Source: CAD feature listing. Evaluate the final solid. Frame: model axes, mm. A direction names the side the tool comes from. Give positions to 0.01 mm unless a question says otherwise; leave off trailing zeros. Write each loop counter-clockwise with the first axis right and the second up, starting at its lowest first coordinate (ties: lowest second). Pieces come first, ordered by that corner, then holes. Notation, with made-up numbers: M -8,79 L 11,79 A8 cw 11,84 Z; hole C 35,43.5 d2. An arc over 180 degrees is marked long. Return JSON: item names as keys, results as strings.
```python
from build123d import *

# Parameters (mm, degrees)
F1_DEPTH = 360.3625
F2_R     = 3.175
F3_DEPTH = 9.525


with BuildPart() as f1:
    # F0 (on Front) → F1 (new body)
    with BuildSketch(Plane.XZ):
        Polygon((3.666174, 6.35), (-3.666174, 6.35), (-7.332348, 0), (-3.666174, -6.35), (3.666174, -6.35), (7.332348, 0), align=None)
    extrude(amount=F1_DEPTH)

    # F2 (on face) → F3 (cut)
    with BuildSketch(Plane(origin=(0, 0, 0), x_dir=(-1, 0, 0), z_dir=(0, 1, 0))):
        Circle(F2_R)
    extrude(amount=-F3_DEPTH, mode=Mode.SUBTRACT)


solid = f1.part
```
1) Cut plane A-A, the plane y = -59. Return the cut outline in (x, z), then the cut area to 3 significant figures.
Numbers:
{"outline": "M -7.33,0 L -3.67,-6.35 L 3.67,-6.35 L 7.33,0 L 3.67,6.35 L -3.67,6.35 Z", "area": "140 mm²"}
2) Line query: line 1 (Z direction, x = 0, y = -7.5) (3 decimals); line 2 (Y direction, x = 0, z = -0.25) (1 decimal); line 3 (X direction, y = -53.5, z = 4.25). Output: solid intervals per line, ascending. Write a range as [from, to].
Numbers:
{"line 1": "z = [-6.35, -3.175], [3.175, 6.35]", "line 2": "y = [-360.4, -9.5]", "line 3": "x = [-4.88, 4.88]"}
3) Set-up query: faces 1 (the face through (-5.474, -177.659, 3.219)), 2 (the face through (0.69, -4.7, -3.1)). Return all of +Z, -Z, +X, -X, +Y, -Y with unobstructed straight access to the full face (end or side cutting, diameter ignored); none if empty.
Numbers:
{"face 1": "+Z, -X, +Y, -Y", "face 2": "+Y"}
4) Contact query for flat-ended pins moving along their axis: pin 1 Ø3 at (y, z) = (-246.5, -5) entering from +X; pin 2 Ø1 at (y, z) = (-74.5, 2.5) entering from -X; pin 3 Ø5 at (y, z) = (-70, -4) entering from +X. Output: stop coordinate, or through.
Numbers:
{"pin 1": "stops at x = 5.31", "pin 2": "stops at x = -6.18", "pin 3": "stops at x = 6.47"}
5) Draft query along X for faces 3 (the face through (0, -178, 6.35)), 4 (the face through (0, -9.525, 0)), 5 (the face through (5.525, -177.659, 3.131)). Return one class per face: released by +X, released by -X, zero draft, split by the parting line, or undercut.
Numbers:
{"face 3": "zero draft", "face 4": "undercut", "face 5": "released by +X"}
